Drawing for the job (mm, zero at the part's lowest x, y, z). A direction names the side the tool comes from. Coordinates: 2 decimals unless noted, no trailing zeros. Write each loop counter-clockwise with the first axis right and the second up, starting at its lowest first coordinate (ties: lowest second). Pieces come first, ordered by that corner, then holes.
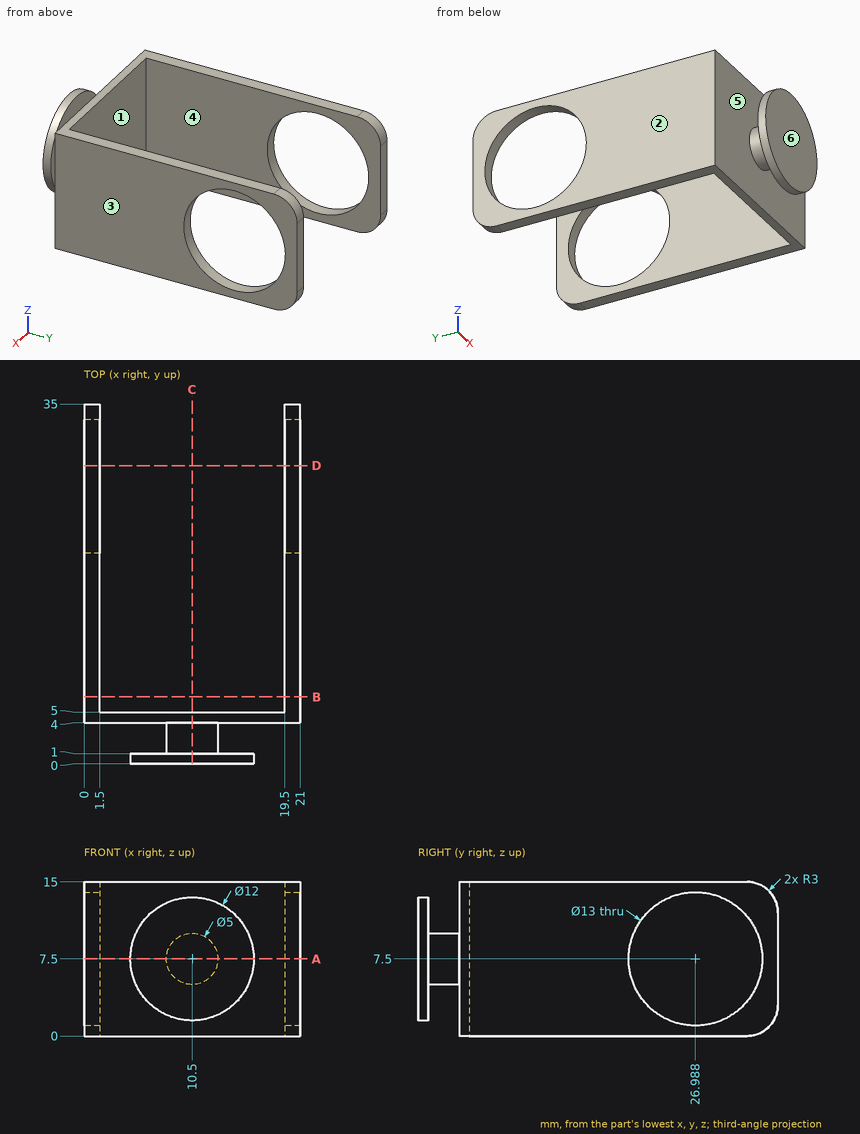
Item 1: Two-plate mould, pull along X, no slides. Class the marked faces 1, 2 and 3: +X half, -X half, draft (parallel to the pull), parting line (faces both ways), or undercut.
Item 2: Wall check: line 1 along Y through (x, z) = (1.1, 7.5); line 2 along X through (y, z) = (17.5, 5.5); line 3 along Y through (x, z) = (12, 10). Give the ranges that are in metal, low to high.
Item 3: Saw through at D-D, the plane y = 29. Write the cut outline in (x, z).
Item 4: Which spindle directions (+Z, -Z, +X, -X, +Y, -Y) get a long thin tool onto all of the face, cutting with end or side? Do the marked faces 4, 5 and 6. Say none if no direction does.
Item 5: Saw through at A-A, the plane z = 7.5. Write the cut outline in (x, y).
Item 6: Flat gauge pins, fed straight in: pin 1 Ø3 at (x, y) = (2.5, 8) entering from +Z; pin 2 Ø4 at (x, z) = (15.5, 6) entering from +Y. Where does each tip first touch, or does it go through?
Item 7: Saw through at C-C, the plane x = 10.5. Write the cut outline in (y, z), and give its area (3 significant figures).
Item 8: Saw through at B-B, the plane y = 6.5. Write the cut outline in (x, z).
Working result:
1. face 1: undercut
1. face 2: -X half
1. face 3: +X half
2. line 1: y = 4 to 20.49, 33.49 to 35
2. line 2: x = 0 to 1.5, 19.5 to 21
2. line 3: y = 0 to 1, 4 to 5
3. outline: (0, 0) - (1.5, 0) - (1.5, 1.32) - (0, 1.32) - close; (0, 13.68) - (1.5, 13.68) - (1.5, 15) - (0, 15) - close; (19.5, 0) - (21, 0) - (21, 1.32) - (19.5, 1.32) - close; (19.5, 13.68) - (21, 13.68) - (21, 15) - (19.5, 15) - close
4. face 4: +Z, -Z, +Y
4. face 5: none
4. face 6: +Z, -Z, +X, -X, -Y
5. outline: (0, 4) - (8, 4) - (8, 1) - (4.5, 1) - (4.5, 0) - (16.5, 0) - (16.5, 1) - (13, 1) - (13, 4) - (21, 4) - (21, 20.49) - (19.5, 20.49) - (19.5, 5) - (1.5, 5) - (1.5, 20.49) - (0, 20.49) - close; (0, 33.49) - (1.5, 33.49) - (1.5, 35) - (0, 35) - close; (19.5, 33.49) - (21, 33.49) - (21, 35) - (19.5, 35) - close
6. pin 1: stops at z = 15
6. pin 2: stops at y = 5
7. outline: (0, 1.5) - (1, 1.5) - (1, 5) - (4, 5) - (4, 0) - (5, 0) - (5, 15) - (4, 15) - (4, 10) - (1, 10) - (1, 13.5) - (0, 13.5) - close
7. area: 42.0 mm2
8. outline: (0, 0) - (1.5, 0) - (1.5, 15) - (0, 15) - close; (19.5, 0) - (21, 0) - (21, 15) - (19.5, 15) - close
